```python
from build123d import *

# Parameters (mm, degrees)
SKETCH3_W          = 1.5
SKETCH3_H          = 1
SKETCH3_W_2        = 1
SKETCH3_H_2        = 1.5
CUT_EXTRUDE1_DEPTH = 1.5


with BuildPart() as part:
    # Sketch2 → Revolve1 (revolve)
    with BuildSketch(Plane.XY, mode=Mode.PRIVATE) as revolve1_sk:
        Polygon((0, 2.5), (3.65, 2.5), (3.65, 1.5), (2, 0), (2, -52.5), (0, -52.5), align=None)
    revolve(revolve1_sk.sketch.rotate(Axis((0, 27.929971315, 0), (0, -1, 0)), 180), axis=Axis((0, 27.929971315, 0), (0, -1, 0)))

    # Sketch3 → Cut-Extrude1 (cut)
    with BuildSketch(Plane(origin=(0, 2.5, 0), x_dir=(1, 0, 0), z_dir=(0, 1, 0))):
        with Locations((1.25, 0)):
            Rectangle(SKETCH3_W, SKETCH3_H)
        with Locations((0, 1.25)):
            Rectangle(SKETCH3_W_2, SKETCH3_H_2)
        with Locations((-1.25, 0)):
            Rectangle(SKETCH3_W, SKETCH3_H)
        Rectangle(SKETCH3_W_2, SKETCH3_H)
        with Locations((0, -1.25)):
            Rectangle(SKETCH3_W_2, SKETCH3_H_2)
    extrude(amount=-CUT_EXTRUDE1_DEPTH, mode=Mode.SUBTRACT)


solid = part.part
```
Source: CAD feature listing. Evaluate the final solid. Frame: model axes, mm. A direction names the side the tool comes from. Give positions to 0.01 mm unless a question says otherwise; leave off trailing zeros. Write each loop counter-clockwise with the first axis right and the second up, starting at its lowest first coordinate (ties: lowest second). Pieces come first, ordered by that corner, then holes. Notation, with made-up numbers: (-3, 85.5) - (21, 85.5) arc R17 cw to (21, 89.5) - close; hole circle Ø7 at (82.5, -16.75). An arc over 180 degrees is marked (long way). One line per item, written item: value. Start each with the question number.
Q1. First-contact query: pin 1 Ø1 at (x, y) = (1, -12) entering from +Z; pin 2 Ø1.6 at (y, z) = (2, -1) entering from -X; pin 3 Ø0.8 at (y, z) = (2, 1) entering from +X; pin 4 Ø3 at (x, z) = (-1, 0) entering from +Y. Flat tips, straight axial feed; report the tip coordinate or a pass-through.
Q2. Section query B-B, the plane y = -6.5. Return the cut outline in (x, z).
Q3. Set-up query: faces 4 (the face through (0, -27, 2)), 5 (the face through (1, 2.5, 1)), 6 (the face through (0, 2, 2)). Return all of +Z, -Z, +X, -X, +Y, -Y with unobstructed straight access to the full face (end or side cutting, diameter ignored); none if empty.
Q4. Section query A-A, the plane x = 0. Return the cut outline in (y, z).
Q5. Material intervals for probe 1 along Y at (x, z) = (0.75, -3); probe 2 along Y at (x, z) = (0, 0.5); probe 3 along Z at (x, y) = (1.75, -35.5), sorted ascending. Write a range as from..to.
Q6. Draft query along Z for faces 1 (the face through (-3.48, 1.99, -1.1)), 2 (the face through (0, 1, 0)), 3 (the face through (0, -52.5, 0)). Return one class per face: +Z half, -Z half, draft (parallel to the pull), parting line (faces both ways), or undercut.
Answer:
1. pin 1: stops at z = 1.94
1. pin 2: stops at x = -3.64
1. pin 3: stops at x = 3.6
1. pin 4: stops at y = 2.5
2. outline: circle Ø4 at (0, 0)
3. face 4: -Y
3. face 5: +Z, -Z, +X, -X, +Y
3. face 6: +Y
4. outline: (-52.5, -2) - (0, -2) - (1.5, -3.65) - (2.5, -3.65) - (2.5, -2) - (1, -2) - (1, 2) - (2.5, 2) - (2.5, 3.65) - (1.5, 3.65) - (0, 2) - (-52.5, 2) - close
5. probe 1: y = 0.99..2.5
5. probe 2: y = -52.5..1
5. probe 3: z = -0.97..0.97
6. face 1: parting line
6. face 2: undercut
6. face 3: draft
